```python
from build123d import *

# Parameters (mm, degrees)
EXTRUDE_2_DEPTH = 10


with BuildPart() as part:
    # 草图3 → 凸台-拉伸2 (new body)
    with BuildSketch(Plane(origin=(0, 0, 0), x_dir=(1, 0, 0), z_dir=(0, 1, 0))):
        with BuildLine():
            Line((0, 110), (-4, 110))
            Line((-4, 110), (-4, 99.919967974))
            ThreePointArc((-4, 99.919967974), (-70.710678119, 70.710678119), (-99.919967974, 4))
            Line((-99.919967974, 4), (-110, 4))
            Line((-110, 4), (-110, 0))
            Line((-110, 0), (-110, -4))
            Line((-110, -4), (-99.919967974, -4))
            ThreePointArc((-99.919967974, -4), (-70.710678119, -70.710678119), (-4, -99.919967974))
            Line((-4, -99.919967974), (-4, -110))
            Line((-4, -110), (0, -110))
            Line((0, -110), (4, -110))
            Line((4, -110), (4, -99.919967974))
            ThreePointArc((4, -99.919967974), (70.710678119, -70.710678119), (99.919967974, -4))
            Line((99.919967974, -4), (110, -4))
            Line((110, -4), (110, 0))
            Line((110, 0), (110, 4))
            Line((110, 4), (99.919967974, 4))
            ThreePointArc((99.919967974, 4), (70.710678119, 70.710678119), (4, 99.919967974))
            Line((4, 99.919967974), (4, 110))
            Line((4, 110), (0, 110))
        make_face()
    extrude(amount=EXTRUDE_2_DEPTH)


solid = part.part
```
CAD build for the part. Positions are in the model's coordinates, mm. A direction names the side the tool comes from. Give positions to 0.01 mm unless a question says otherwise; leave off trailing zeros. Loops run counter-clockwise (first coordinate to the right, second up) from the corner with the lowest first, then second, coordinate; pieces in that order, holes last. Notation, with made-up numbers: (-1, 22) -> (5, 22) arc R37 cw to (5, 60) -> close; hole circle Ø10 at (-17, -12). An arc over 180 degrees is marked (long way). Use a Markdown table: item, result.
1. Flat gauge pins, fed straight in: pin 1 (2 mm diameter, centred on y = 7, z = -87.5, fed in from +X); pin 2 (2 mm diameter, centred on x = 31.5, z = 59, fed in from -Y); pin 3 (3 mm diameter, centred on y = 9, z = 69.5, fed in from +X); pin 4 (5 mm diameter, centred on x = 107, y = 3.5, fed in from +Z). Where does each tip first touch, or does it go through?
Check result:
| item | result |
|---|---|
| pin 1 | stops at x = 50.18 |
| pin 2 | stops at y = 0 |
| pin 3 | stops at x = 73.32 |
| pin 4 | stops at z = 4 |
2. Slice it at B-B (z = 12.5). List the corners of the cut face in (x, y), plus the area to 3 significant figures.
Check result:
| item | result |
|---|---|
| outline | (-99.22, 0) -> (99.22, 0) -> (99.22, 10) -> (-99.22, 10) -> close |
| area | 1,980 mm^2 |
3. Slice it at A-A (y = 3.5). List the corners of the cut face in (x, z), plus the area to 3 significant figures.
Check result:
| item | result |
|---|---|
| outline | (-110, -4) -> (-99.92, -4) arc R100 ccw to (-4, -99.92) -> (-4, -110) -> (4, -110) -> (4, -99.92) arc R100 ccw to (99.92, -4) -> (110, -4) -> (110, 4) -> (99.92, 4) arc R100 ccw to (4, 99.92) -> (4, 110) -> (-4, 110) -> (-4, 99.92) arc R100 ccw to (-99.92, 4) -> (-110, 4) -> close |
| area | 31,700 mm^2 |
4. Wall check: L1, parallel to Z at x = -55, y = 7.5; L2, parallel to X at y = 8.75, z = -85; L3, parallel to X at y = 8.5, z = 101. Give the ranges that are in metal, low to high. Write a range as [from, to].
Check result:
| item | result |
|---|---|
| L1 | z = [-83.52, 83.52] |
| L2 | x = [-52.68, 52.68] |
| L3 | x = [-4, 4] |
5. Which spindle directions (+Z, -Z, +X, -X, +Y, -Y) get a long thin tool onto all of the face, cutting with end or side? Do faces 1 (the flat face through (4, 5, 105)), 2 (the flat face through (4, 5, -105)), 3 (the flat face through (-105, 5, -4)). Say none if no direction does.
Check result:
| item | result |
|---|---|
| face 1 | +Z, +X, +Y, -Y |
| face 2 | -Z, +X, +Y, -Y |
| face 3 | -Z, -X, +Y, -Y |
6. Slice it at C-C (x = 19). List the corners of the cut face in (y, z), plus the area to 3 significant figures.
Check result:
| item | result |
|---|---|
| outline | (0, -98.18) -> (10, -98.18) -> (10, 98.18) -> (0, 98.18) -> close |
| area | 1,960 mm^2 |
